Autodesk Fusion 360 part; units mm, degrees
sketch "Sketch1" plane through (0, 0, 0) normal (0, 1, 0) x (1, 0, 0)
  line L0 (72, -50) -> (-1, -50)
  line L1 (1.5, -2.5) -> (69.5, -2.5)
  line L2 (69.5, -47.5) -> (1.5, -47.5)
  circle A0 centre (5.5, -5.25) radius 1.5
  circle A1 centre (5.5, -44.75) radius 1.5
  circle A2 centre (46, -5.25) radius 1.5
  circle A3 centre (46, -44.75) radius 1.5
  line L3 (46, -7.5) -> (5.25, -7.5)
  line L4 (5.25, -7.5) -> (5.25, -42.5)
  line L5 (5.25, -42.5) -> (46, -42.5)
  line L6 (46, -42.5) -> (46, -7.5)
  line L7 (46, -7.5) -> (5.25, -42.5) construction
  line L8 (5.25, -7.5) -> (46, -42.5) construction
  line L9 (72, 0) -> (-1, 0)
  line L10 (-1, 39.9342) -> (-1, -50)
  line L11 (1.5, -47.5) -> (1.5, -2.5)
  line L12 (67.25, -14.5) -> (48.25, -14.5)
  line L13 (48.25, -14.5) -> (48.25, -40.5)
  line L14 (48.25, -40.5) -> (67.25, -40.5)
  line L15 (67.25, -40.5) -> (67.25, -14.5)
  line L16 (67.25, -14.5) -> (48.25, -40.5) construction
  line L17 (48.25, -14.5) -> (67.25, -40.5) construction
  line L18 (67.25, -14.5) -> (60.25, -14.5)
  line L19 (69.5, -2.5) -> (69.5, -47.5)
  line L20 (72, 0) -> (72, -50)
  circle A4 centre (60.25, -25.5) radius 3.875
  line L21 (48.25, -14.5) -> (50.75, -14.5)
  circle A5 centre (50.75, -20.5) radius 1.5
  circle A6 centre (50.75, -34.5) radius 1.5
  point P0 (25.625, -25)
  point P1 (57.75, -27.5)
  dimension "d10" = 3
  dimension "d12" = 35
  dimension "d15" = 19
  dimension "d19" = 26
  dimension "d20" = 2.5
  dimension "d21" = 40.75
  dimension "d22" = 4
  dimension "d30" = 7.75
  dimension "d31" = 2.5
  dimension "d32" = 6
  dimension "d34" = 3
  dimension "d35" = 3
  dimension "d36" = 7
  dimension "d37" = 11
extrude "Extrude1" add sketch "Sketch1" against normal blind 3 contours L1 L2 L11 L19 | L12 L13 L14 L15 L18 L21
extrude "Extrude2" add sketch "Sketch1" against normal blind 20 contours L0 L9 L10 L20
sketch "Sketch2" plane through (0, 0, 0) normal (0, 1, 0) x (1, 0, 0)
  line L0 (72, 0) -> (72, -50)
  line L1 (72, -25) -> (72, -27.75)
  line L2 (72, -27.75) -> (75.5, -27.75)
  line L3 (77.5, -25.75) -> (77.5, -24.25)
  line L4 (75.5, -22.25) -> (72, -22.25)
  line L5 (72, -22.25) -> (72, -27.75)
  circle A0 centre (74.75, -25) radius 1.5
  line L6 (72, 0) -> (-1, 0)
  line L7 (35.5, 0) -> (35.5, -15)
  arc A1 (77.5, -24.25) -> (75.5, -22.25) centre (75.5, -24.25) ccw
  arc A2 (75.5, -27.75) -> (77.5, -25.75) centre (75.5, -25.75) ccw
  circle A3 centre (-3.75, -25) radius 1.5
  arc A4 (-6.5, -25.75) -> (-4.5, -27.75) centre (-4.5, -25.75) ccw
  arc A5 (-4.5, -22.25) -> (-6.5, -24.25) centre (-4.5, -24.25) ccw
  line L8 (-1, -22.25) -> (-1, -27.75)
  line L9 (-4.5, -22.25) -> (-1, -22.25)
  line L10 (-6.5, -25.75) -> (-6.5, -24.25)
  line L11 (-1, -27.75) -> (-4.5, -27.75)
  line L12 (-1, 0) -> (-1, -50)
  line L13 (-1, -25) -> (-1, -27.75)
  point P0 (77.5, -27.75)
  point P1 (-6.5, -27.75)
  dimension "d45" = 5.5
  dimension "d46" = 5.5
  dimension "d47" = 3
  dimension "d48" = 15
  dimension "d49" = 2
  dimension "d50" = 2
extrude "Extrude3" add sketch "Sketch2" against normal blind 20 contours A4 A5 L8 L9 L10 L11 L12 L13
extrude "Extrude4" cut sketch "Sketch2" against normal blind 17 contours A4 A5 L8 L9 L10 L11 L12 L13
extrude "Extrude5" add sketch "Sketch2" against normal blind 20 contours L0 L1 L2 L3 L4 L5 A1 A2
extrude "Extrude6" cut sketch "Sketch2" against normal blind 17 contours L0 L1 L2 L3 L4 L5 A1 A2
Source: CAD feature listing. Evaluate the final solid. Frame: model axes, mm. A direction names the side the tool comes from. Give positions to 0.01 mm unless a question says otherwise; leave off trailing zeros. Order: outer loops, then holes, each group sorted by start corner. A loop starts at its lowest first (then second) coordinate and runs counter-clockwise, first axis right, second up.
(1) Section query A-A (x = 60.25). Return the cut outline in (y, z) (3 decimals).
(2) Section query C-C (y = -18). Return the cut outline in (x, z), plus the area to 3 significant figures.
(3) Section query D-D (z = 15). Return the cut outline in (x, y), plus the area to 3 significant figures.
(4) Contact query for flat-ended pins moving along their axis: P1, Ø3, axis at x = 76, z = 26, coming from the +Y side; P2, Ø10, axis at y = -5.5, z = 30.5, coming from the -X side; P3, Ø1.5, axis at y = -10.5, z = 31.5, coming from the +X side. Output: stop coordinate, or through.
(5) Access query for faces 1 (the face through (36, -11, 47.5)), 2 (the face through (5.25, -1, 25)), 3 (the face through (-2.6, -17, 23.7)). Directions: +Z, -Z, +X, -X, +Y, -Y. A direction counts if a zero-diameter tool reaches every point of the face in a straight line with its end or side. Return the directions, or none.
(6) Pull-direction query (Z, two-part tool) for faces 4 (the face through (77.5, -18, 25)), 5 (the face through (74, -18, 27.75)), 6 (the face through (26, -1, 7.5)); classes: +Z half, -Z half, draft (parallel to the pull), parting line (faces both ways), or undercut.
(7) Material intervals for line 1 along X through (y, z) = (-0.7, 20.5); line 2 along Z through (x, y) = (50.75, -1.3); line 3 along X through (y, z) = (-2.15, 44.75), sorted ascending.
(8) Section query B-B (z = 44.75). Return the cut outline in (x, y), plus the area to 3 significant figures.
Outcome:
1. outline: (-20, 0) - (0, 0) - (0, 21.625) - (-3, 21.625) - (-3, 2.5) - (-20, 2.5) - close; (-20, 47.5) - (-3, 47.5) - (-3, 29.375) - (0, 29.375) - (0, 50) - (-20, 50) - close
2. outline: (-6.5, 24.25) arc R2 ccw to (-4.5, 22.25) - (-1, 22.25) - (-1, 0) - (72, 0) - (72, 22.25) - (75.5, 22.25) arc R2 ccw to (77.5, 24.25) - (77.5, 25.75) arc R2 ccw to (75.5, 27.75) - (72, 27.75) - (72, 50) - (-1, 50) - (-1, 27.75) - (-4.5, 27.75) arc R2 ccw to (-6.5, 25.75) - close; hole circle Ø3 at (-3.75, 25); hole (1.5, 2.5) - (69.5, 2.5) - (69.5, 47.5) - (1.5, 47.5) - close; hole circle Ø3 at (74.75, 25)
2. area: 633 mm2
3. outline: (-1, -20) - (1.5, -20) - (1.5, -3) - (5.25, -3) - (5.25, 0) - (-1, 0) - close; (46, -3) - (69.5, -3) - (69.5, -20) - (72, -20) - (72, 0) - (46, 0) - close
3. area: 182 mm2
4. P1: stops at y = -17
4. P2: stops at x = -1
4. P3: stops at x = 72
5. face 1: -Y
5. face 2: +Y, -Y
5. face 3: +Z, -Z, -X, +Y
6. face 4: draft
6. face 5: +Z half
6. face 6: undercut
7. line 1: x = -1 to 5.25, 46 to 49.25, 52.25 to 72
7. line 2: z = 0 to 19, 22 to 33, 36 to 50
7. line 3: x = -1 to 4, 7 to 44.5, 47.5 to 72
8. outline: (-1, -20) - (1.5, -20) - (1.5, -3) - (4, -3) - (4, 0) - (-1, 0) - close; (7, -3) - (44.5, -3) - (44.5, 0) - (7, 0) - close; (47.5, -3) - (69.5, -3) - (69.5, -20) - (72, -20) - (72, 0) - (47.5, 0) - close
8. area: 286 mm2
